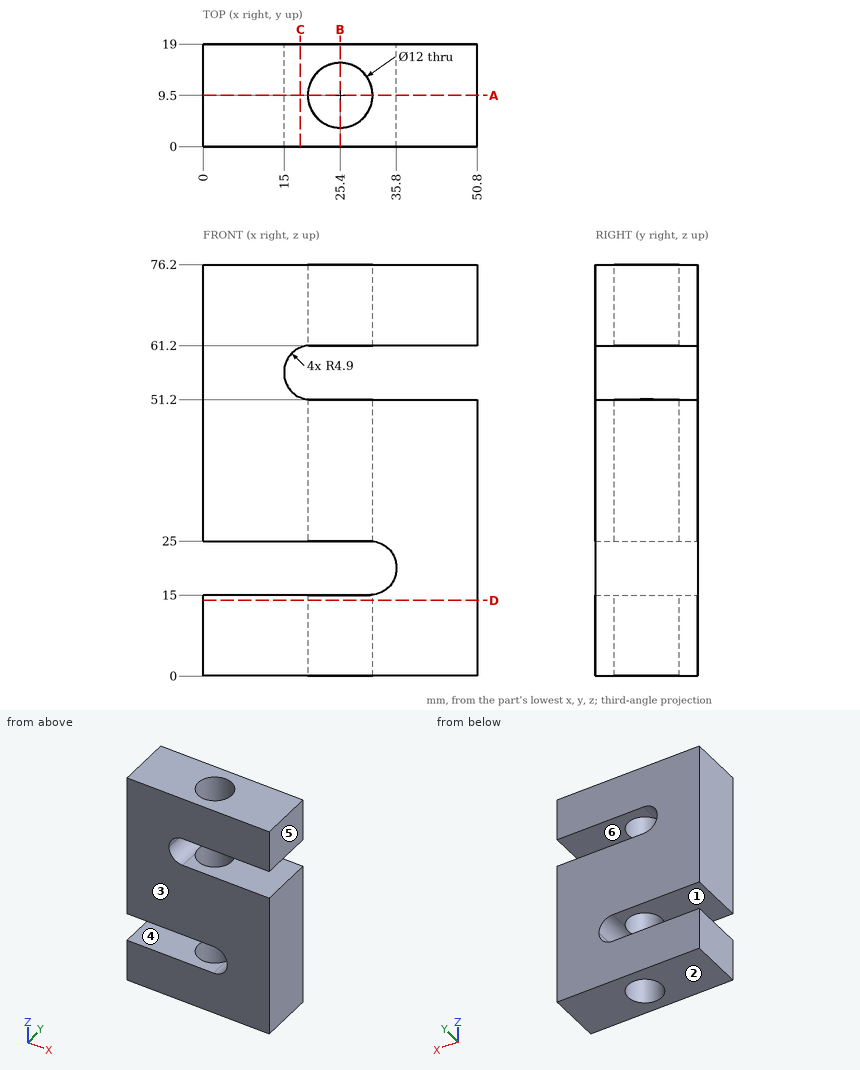
Input: dimensioned drawing with shaded views. Units: mm. Origin: part minimum x, y, z. A direction names the side the tool comes from. Round coordinates to 2 decimals unless told otherwise and drop trailing zeros. Loops run counter-clockwise (first coordinate to the right, second up) from the corner with the lowest first, then second, coordinate; pieces in that order, holes last. Notation, with made-up numbers: (-35.75, -27) -> (-14.75, -27) arc R20 cw to (-14.75, -15) -> close; hole circle Ø4 at (-36, 40). An arc over 180 degrees is marked (long way). Answer as a JSON object with one key per item and string values. Group by question number.
1) Reachability of the marked faces 4, 5 and 6 from +Z, -Z, +X, -X, +Y, -Y: full face, straight path, thin tool, end or side. Return the list, or none.
2) Section query D-D on z = 14. Output: boundary loops of the cut face in (x, y), plus the area to 3 significant figures.
3) Section query B-B on x = 25.4. Output: boundary loops of the cut face in (y, z), plus the area to 3 significant figures.
4) Pin query (flat end, axial travel): pin 1 (9.5 mm diameter, centred on x = 25.4, y = 9.5, fed in from -Z). Return the tip coordinate at first contact, or that it passes through.
5) Draft query along Z for the marked faces 1, 2 and 3. Return one class per face: +Z half, -Z half, draft (parallel to the pull), parting line (faces both ways), or undercut.
6) Section query A-A on y = 9.5. Output: boundary loops of the cut face in (x, z), plus the area to 3 significant figures.
7) Ray query, L1, parallel to Z at x = 24.5, y = 18.25; L2, parallel to Z at x = 7, y = 11; L3, parallel to Z at x = 44, y = 8.25. Return the intervals inside material, ascending.
8) Section query C-C on x = 18. Output: boundary loops of the cut face in (y, z), plus the area to 3 significant figures.
Reply:
{
 "1": {"face 4": "-X, +Y, -Y", "face 5": "+Z, -Z, +X, +Y, -Y", "face 6": "+X, +Y, -Y"},
 "2": {"outline": "(0, 0) -> (50.8, 0) -> (50.8, 19) -> (0, 19) -> close; hole circle Ø12 at (25.4, 9.5)", "area": "852 mm2"},
 "3": {"outline": "(0, 0) -> (3.5, 0) -> (3.5, 15) -> (0, 15) -> close; (0, 25) -> (3.5, 25) -> (3.5, 51.2) -> (0, 51.2) -> close; (0, 61.2) -> (3.5, 61.2) -> (3.5, 76.2) -> (0, 76.2) -> close; (15.5, 0) -> (19, 0) -> (19, 15) -> (15.5, 15) -> close; (15.5, 25) -> (19, 25) -> (19, 51.2) -> (15.5, 51.2) -> close; (15.5, 61.2) -> (19, 61.2) -> (19, 76.2) -> (15.5, 76.2) -> close", "area": "393 mm2"},
 "4": {"pin 1": "passes through"},
 "5": {"face 1": "undercut", "face 2": "-Z half", "face 3": "draft"},
 "6": {"outline": "(0, 0) -> (19.4, 0) -> (19.4, 15) -> (0, 15) -> close; (0, 25) -> (19.4, 25) -> (19.4, 51.23) arc R4.9 cw to (15, 56.1) -> (15, 56.3) arc R4.9 cw to (19.4, 61.17) -> (19.4, 76.2) -> (0, 76.2) -> close; (31.4, 0) -> (50.8, 0) -> (50.8, 51.2) -> (31.4, 51.2) -> (31.4, 24.97) arc R4.9 cw to (35.8, 20.1) -> (35.8, 19.9) arc R4.9 cw to (31.4, 15.03) -> close; (31.4, 61.2) -> (50.8, 61.2) -> (50.8, 76.2) -> (31.4, 76.2) -> close", "area": "2,500 mm2"},
 "7": {"L1": "z = 0 to 15, 25 to 51.2, 61.2 to 76.2", "L2": "z = 0 to 15, 25 to 76.2", "L3": "z = 0 to 51.2, 61.2 to 76.2"},
 "8": {"outline": "(0, 0) -> (19, 0) -> (19, 15) -> (0, 15) -> close; (0, 25) -> (19, 25) -> (19, 51.58) -> (0, 51.58) -> close; (0, 60.82) -> (19, 60.82) -> (19, 76.2) -> (0, 76.2) -> close", "area": "1,080 mm2"}
}
